Could you check a few things on this model? Use its own coordinates, in mm. Face numbers are marked on the shaded views. Give positions to 0.01 mm unless a question says otherwise; leave off trailing zeros. Write each loop counter-clockwise with the first axis right and the second up, starting at its lowest first coordinate (ties: lowest second). Pieces come first, ordered by that corner, then holes. Notation, with made-up numbers: M 76.25,-11.75 L 123.25,-11.75 A20 ccw 123.25,-5.75 Z; hole C -17,7 d6. An arc over 180 degrees is marked long. Use one line per item in the form item = value.
from build123d import *

# Parameters (mm, degrees)
F1_DEPTH = 125.1
F2_W     = 44
F2_H     = 7.301
F3_DEPTH = 125.1
F4_R     = 8
F5_DEPTH = 4


with BuildPart() as f1:
    # F0 (on Front) → F1 (new body)
    with BuildSketch(Plane.XZ):
        with BuildLine():
            ThreePointArc((-34.5, 0), (0, 34.5), (34.5, 0))
            Line((34.5, 0), (42.5, 0))
            ThreePointArc((42.5, 0), (0, 42.5), (-42.5, 0))
            Line((-42.5, 0), (-34.5, 0))
        make_face()
    extrude(amount=F1_DEPTH)

    # F2 (on Front) → F3 (cut)
    with BuildSketch(Plane.XZ):
        with Locations((0, 42)):
            Rectangle(F2_W, F2_H)
    extrude(amount=F3_DEPTH, mode=Mode.SUBTRACT)

    # F4 (on face) → F5 (cut)
    with BuildSketch(Plane.XY.offset(38.3495)):
        with Locations((0, -62.5)):
            Circle(F4_R)
    extrude(amount=-F5_DEPTH, mode=Mode.SUBTRACT)


solid = f1.part
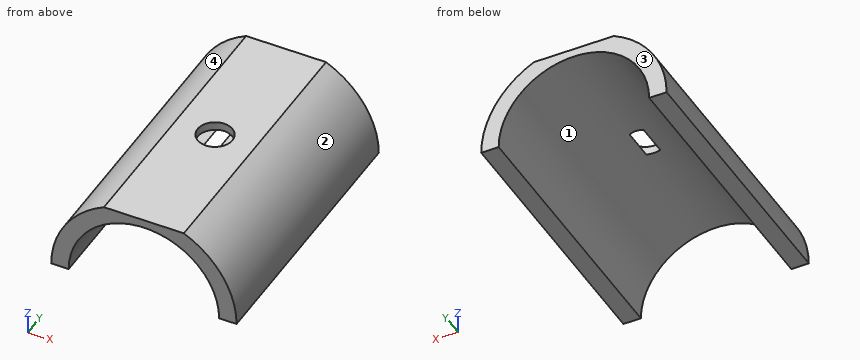
1) For pin 1 Ø6 at (y, z) = (-46.5, 34) entering from +X; pin 2 Ø1.5 at (y, z) = (-66, 6) entering from +X; pin 3 Ø12 at (y, z) = (-53, 27) entering from +X, each with a flat end and sliding along its axis, tell me the tip position at first contact or that it passes through.
Checked values:
pin_1 = 29.07
pin_2 = 42.17
pin_3 = 36.95
2) I want a section at D-D, the plane y = -24. Please give me the cut outline in (x, z), plus the area to 3 significant figures.
Checked values:
outline = M -42.5,0 L -34.5,0 A34.5 cw 34.5,0 L 42.5,0 A42.5 ccw 18.32,38.35 L -18.32,38.35 A42.5 ccw Z
area = 865 mm2
3) Thinking about a two-plate mould opening in X: for the marked faces 1, 2, 3 and 4, which applies, released by +X, released by -X, zero draft, split by the parting line, or undercut?
Checked values:
face_1 = undercut
face_2 = released by +X
face_3 = zero draft
face_4 = released by -X
4) I want a section at C-C, the plane z = 21.5. Please give me the cut outline in (x, y), plus the area to 3 significant figures.
Checked values:
outline = M -36.66,-125.1 L -26.98,-125.1 L -26.98,0 L -36.66,0 Z; M 26.98,-125.1 L 36.66,-125.1 L 36.66,0 L 26.98,0 Z
area = 2,420 mm2
5) If I drill on L1, parallel to Y at x = 0, z = 35; L2, parallel to X at y = -6.5, z = 31.5; L3, parallel to X at y = -10.5, z = 20.5, over which ranges is the centre line in solid material (lowest first)?
Checked values:
L1 = -125.1 to -70.5, -54.5 to 0
L2 = -28.53 to -14.07, 14.07 to 28.53
L3 = -37.23 to -27.75, 27.75 to 37.23
6) I want a section at B-B, the plane x = 0. Please give me the cut outline in (y, z).
Checked values:
outline = M -125.1,34.5 L -70.5,34.5 L -70.5,38.35 L -125.1,38.35 Z; M -54.5,34.5 L 0,34.5 L 0,38.35 L -54.5,38.35 Z
7) I want a section at A-A, the plane y = -62.5. Please give me the cut outline in (x, z), plus the area to 3 significant figures.
Checked values:
outline = M -42.5,0 L -34.5,0 A34.5 cw -3.22,34.35 L -8,34.35 L -8,38.35 L -18.32,38.35 A42.5 ccw Z; M 3.22,34.35 A34.5 cw 34.5,0 L 42.5,0 A42.5 ccw 18.32,38.35 L 8,38.35 L 8,34.35 Z
area = 802 mm2
